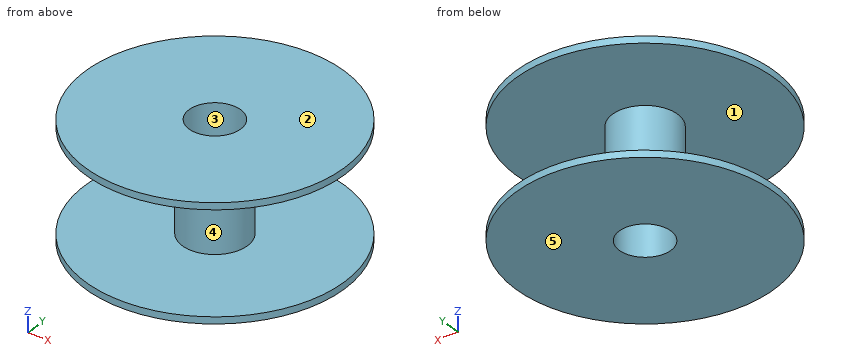
Autodesk Inventor part; units mm, degrees
ref_plane "YZ Plane" through (0, 0, 0) normal (1, 0, 0) x (0, 1, 0)
ref_plane "XZ Plane" through (0, 0, 0) normal (0, 1, 0) x (-1, 0, 0)
ref_plane "XY Plane" through (0, 0, 0) normal (0, 0, 1) x (1, 0, 0)
sketch "Sketch1" plane through (0, 0, 0) normal (0, 0, 1) x (1, 0, 0)
  circle A0 centre (0, 0) radius 95
  circle A1 centre (0, 0) radius 19
  dimension "d0" = 38
  dimension "d2" = 190
extrude "Extrusion1" add sketch "Sketch1" along normal blind 5
sketch "Sketch2" plane through (0, 0, 5) normal (0, 0, 1) x (1, 0, 0)
  circle A0 centre (0, 0) radius 19
  circle A1 centre (0, 0) radius 95
  circle A2 centre (0, 0) radius 24
  dimension "d5" = 5
extrude "Extrusion2" add sketch "Sketch2" along normal blind 75 contours A2
sketch "Sketch3" plane through (0, 0, 80) normal (0, 0, 1) x (1, 0, 0)
  circle A0 centre (0, 0) radius 19
  circle A1 centre (0, 0) radius 24
  circle A2 centre (0, 0) radius 95
extrude "Extrusion3" add sketch "Sketch3" along normal blind 5 contours A1 | A2
properties part number "spool"
Input: part model. Units: mm. Frame: model coordinates. Face numbers are marked on the shaded views. A direction names the side the tool comes from. Coordinates: 2 decimals unless noted, no trailing zeros. Loops run counter-clockwise (first coordinate to the right, second up) from the corner with the lowest first, then second, coordinate; pieces in that order, holes last. Notation, with made-up numbers: M -1,26.5 L 42,26.5 A22 cw 42,46.5 Z; hole C 19.5,-34.75 d11. An arc over 180 degrees is marked long. One line per item, written item: value.
(1) Line query: line 1 along Z through (x, y) = (-86, -22.5); line 2 along Y through (x, z) = (0, 46.5); line 3 along X through (y, z) = (-6, 65). Output: solid intervals per line, ascending. Write a range as from..to.
Filled in:
line 1: 0..5, 80..85
line 2: -24..-19, 19..24
line 3: -23.24..-18.03, 18.03..23.24
(2) Section C-C (z = 45.5). Output: boundary loops of the cut face in (x, y), and give its area (3 significant figures).
Filled in:
outline: C 0,0 d48; hole C 0,0 d38
area: 675 mm^2
(3) Pin query (flat end, axial travel): pin 1 (4 mm diameter, centred on y = 4, z = 28, fed in from +X); pin 2 (12 mm diameter, centred on x = -7, z = 71, fed in from -Y); pin 3 (3 mm diameter, centred on x = -74, y = 44, fed in from -Z). Return the tip coordinate at first contact, or that it passes through.
Filled in:
pin 1: x = 23.92
pin 2: y = -23.98
pin 3: z = 0
(4) Section A-A (x = 0). Output: boundary loops of the cut face in (y, z).
Filled in:
outline: M -95,0 L -19,0 L -19,85 L -95,85 L -95,80 L -24,80 L -24,5 L -95,5 Z; M 19,0 L 95,0 L 95,5 L 24,5 L 24,80 L 95,80 L 95,85 L 19,85 Z
(5) Pull-direction query (X, two-part tool) for the marked faces 3, 4 and 5; classes: +X half, -X half, draft (parallel to the pull), parting line (faces both ways), or undercut.
Filled in:
face 3: undercut
face 4: parting line
face 5: draft
(6) Reachability of the marked faces 1 and 2 from +Z, -Z, +X, -X, +Y, -Y: full face, straight path, thin tool, end or side. Return the list, or none.
Filled in:
face 1: none
face 2: +Z, +X, -X, +Y, -Y
(7) Section D-D (y = 60.5). Output: boundary loops of the cut face in (x, z).
Filled in:
outline: M -73.24,0 L 73.24,0 L 73.24,5 L -73.24,5 Z; M -73.24,80 L 73.24,80 L 73.24,85 L -73.24,85 Z
